```python
from build123d import *

# Parameters (mm, degrees)
F1_DEPTH    = 3.81
F2_W        = 9.0688861602
F2_H        = 3.81
F3_DEPTH    = 6.35
F4_SIZE     = 1.27
F5_W        = 9.0688861602
F5_H        = 3.81
F6_DEPTH    = 5.08
F7_T1_DEPTH = 35.1971853179
F8_R        = 0.9525
F9_DEPTH    = 12.7


# Not quite as in the source:
# - a fillet or chamfer that OpenCascade refuses, or shapes differently, is made with other operations: its cross-section is extruded or revolved along the edge and cut away or added


with BuildPart() as f1:
    # F0 (on Top) → F1 (new body)
    with BuildSketch(Plane.XY):
        with BuildLine():
            Line((4.5344430801, -2.4189800566), (-4.5344430801, -2.4189800566))
            ThreePointArc((-4.5344430801, -2.4189800566), (-11.6244136954, -22.8629027748), (-4.5344430801, -43.306825493))
            Line((-4.5344430801, -43.306825493), (4.5344430801, -43.306825493))
            ThreePointArc((4.5344430801, -43.306825493), (11.6244136954, -22.8629027748), (4.5344430801, -2.4189800566))
        make_face()
    extrude(amount=F1_DEPTH)

    # F2 (on face) → F3 (join)
    with BuildSketch(Plane(origin=(0, -2.4189800566, 0), x_dir=(-1, 0, 0), z_dir=(0, 1, 0))):
        with Locations((0, 1.905)):
            Rectangle(F2_W, F2_H)
    extrude(amount=F3_DEPTH)

    # F4
    f4_edges = [f1.edges().sort_by_distance(p)[0] for p in [
        (0, 3.93102, 0),
    ]]
    chamfer(f4_edges, length=F4_SIZE)

    # F5 (on face) → F6 (join)
    with BuildSketch(Plane.XZ.offset(43.306825493)):
        with Locations((0, 1.905)):
            Rectangle(F5_W, F5_H)
    extrude(amount=F6_DEPTH)

    # F7: chamfer of 5.08 on 1 edges, made by hand

    # F7_s2 → F7_t1 (cut)
    with BuildSketch(Plane.YZ.offset(-17.598592659)):
        Polygon((-43.306825493, 0), (-48.386825493, 5.08), (-48.386825493, 0), align=None)
    extrude(amount=F7_T1_DEPTH, mode=Mode.SUBTRACT)

    # F8 (on face) → F9 (join)
    with BuildSketch(Plane(origin=(0, 3.9310199434, 0), x_dir=(-1, 0, 0), z_dir=(0, 1, 0))):
        with Locations((0, 2.5457337033)):
            Circle(F8_R)
    extrude(amount=F9_DEPTH)


solid = f1.part
```
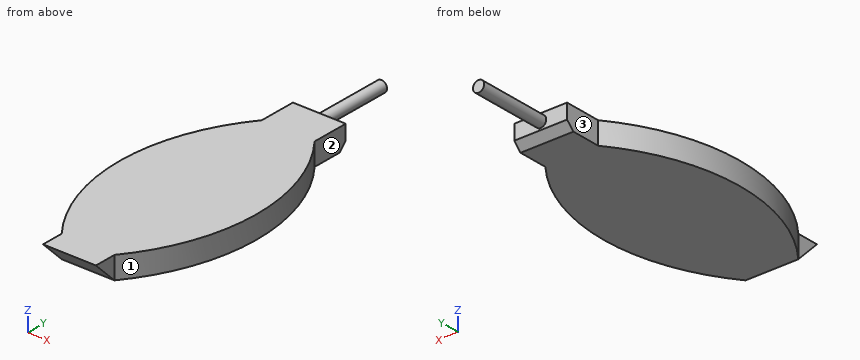
The listing builds one solid part. Answer for the finished solid, in the listing's coordinates (mm). Face numbers are marked on the shaded views. A direction names the side the tool comes from. Round coordinates to 2 decimals unless told otherwise and drop trailing zeros. Loops run counter-clockwise (first coordinate to the right, second up) from the corner with the lowest first, then second, coordinate; pieces in that order, holes last. Notation, with made-up numbers: (-8, -36) -> (4, -36) arc R32 cw to (4, 3) -> close; hole circle Ø11 at (73.5, 51). An arc over 180 degrees is marked (long way). Use one line per item in the form item = value.
1. Flat-ended cylindrical pins translate along their axes: pin 1 Ø2 at (y, z) = (-16.5, 0.5) entering from -X; pin 2 Ø0.8 at (x, z) = (-2, 2.5) entering from +Y; pin 3 Ø2 at (y, z) = (-35.5, 1) entering from +X; pin 4 Ø6 at (x, y) = (-4.5, -25.5) entering from -Z. Find the tip coordinate at first contact, or state that the pin passes through.
Answer key:
pin_1 = -11.19
pin_2 = 3.93
pin_3 = 9.51
pin_4 = 0
2. A tool of negligible diameter and unlimited length cuts with its end or side. For the marked faces 1, 2 and 3, from which of +Z, -Z, +X, -X, +Y, -Y can it reach the whole face along a straight path? Write none if from no direction.
Answer key:
face_1 = +Z, -Z, +X
face_2 = +Z, -Z, +X, +Y
face_3 = +Z, -Z, -X, +Y
3. The part is cut by section A-A on x = 0. Determine the outline of the cut face in (y, z), and give its area (3 significant figures).
Answer key:
outline = (-47.12, 3.81) -> (-43.31, 0) -> (2.66, 0) -> (3.93, 1.27) -> (3.93, 1.59) -> (16.63, 1.59) -> (16.63, 3.5) -> (3.93, 3.5) -> (3.93, 3.81) -> close
area = 211 mm²
4. Find the intervals of material crossed by probe 1 along X at (y, z) = (-1, 3.4); probe 2 along X at (y, z) = (-43, 0.7); probe 3 along Y at (x, z) = (6.75, 1.15), in increasing order. Write a range as [from, to].
Answer key:
probe_1 = [-4.53, 4.53]
probe_2 = [-4.77, 4.77]
probe_3 = [-40.13, -5.6]
5. The part is cut by section B-B on y = -34.5. Determine the outline of the cut face in (x, z).
Answer key:
outline = (-9.51, 0) -> (9.51, 0) -> (9.51, 3.81) -> (-9.51, 3.81) -> close
6. The part is cut by section C-C on x = 6.5. Determine the outline of the cut face in (y, z), and give its area (3 significant figures).
Answer key:
outline = (-40.53, 0) -> (-5.19, 0) -> (-5.19, 3.81) -> (-40.53, 3.81) -> close
area = 135 mm²
